Part print with two shaded views. Sizes in mm from the minimum x, y, z corner. A direction names the side the tool comes from. Coordinates: 2 decimals unless noted, no trailing zeros. Order: outer loops, then holes, each group sorted by start corner. A loop starts at its lowest first (then second) coordinate and runs counter-clockwise, first axis right, second up.
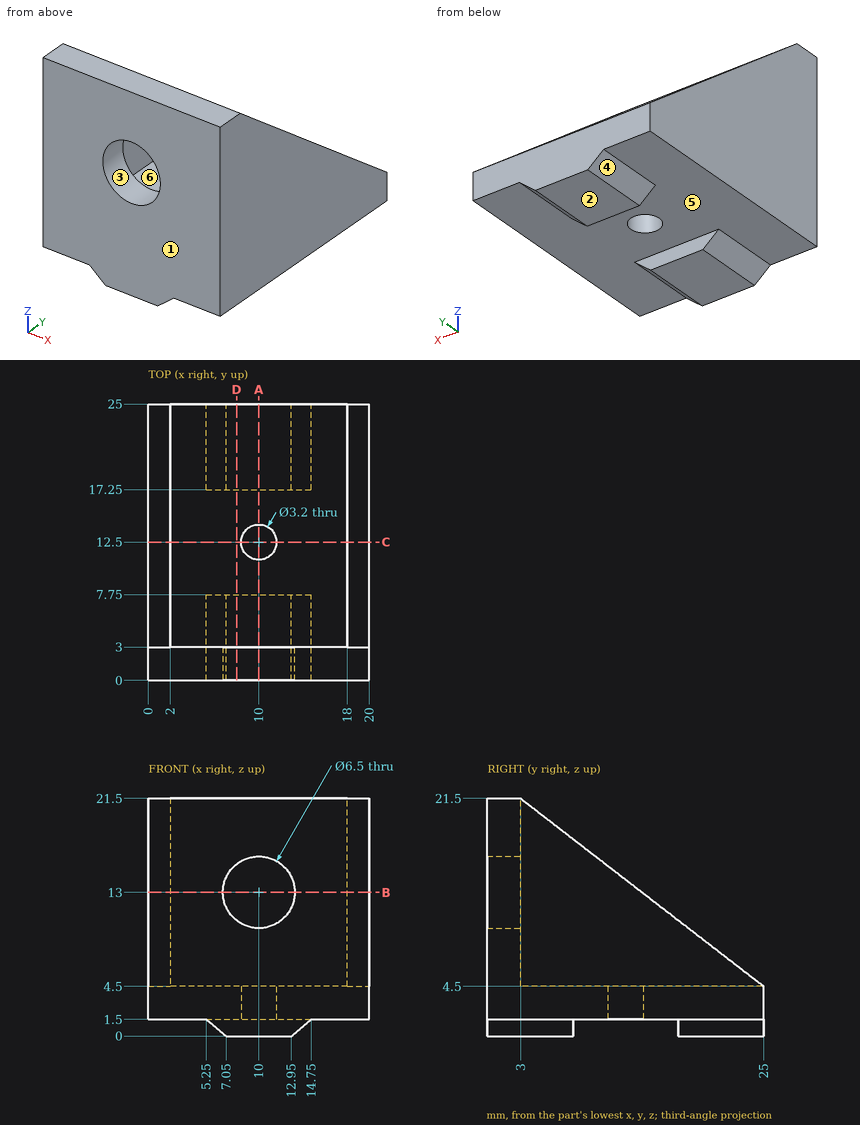
Q1. Pin check, flat tips, straight feed: pin 1 Ø3 at (x, z) = (2, 8.5) entering from -Y; pin 2 Ø8 at (x, y) = (16.5, 11) entering from +Z; pin 3 Ø1.5 at (x, y) = (4, 20) entering from -Z; pin 4 Ø6 at (x, z) = (10, 13) entering from +Y. Stop position of each tip, or through.
Results list:
pin 1: stops at y = 0
pin 2: stops at z = 18.18
pin 3: stops at z = 1.5
pin 4: passes through
Q2. Cut at D-D on x = 8. Write the cut outline in (y, z), and give its area (3 significant figures).
Results list:
outline: (0, 0) - (7.75, 0) - (7.75, 1.5) - (17.25, 1.5) - (17.25, 0) - (25, 0) - (25, 4.5) - (3, 4.5) - (3, 10.44) - (0, 10.44) - close; (0, 15.56) - (3, 15.56) - (3, 21.5) - (0, 21.5) - close
area: 134 mm2
Q3. Cut at B-B on z = 13. Write the cut outline in (x, y).
Results list:
outline: (0, 0) - (6.75, 0) - (6.75, 3) - (2, 3) - (2, 14) - (0, 14) - close; (13.25, 0) - (20, 0) - (20, 14) - (18, 14) - (18, 3) - (13.25, 3) - close
Q4. Wall check: line 1 along Z through (x, y) = (10, 0.95); line 2 along X through (y, z) = (7, 9.25); line 3 along X through (y, z) = (12.5, 3.6). Give the ranges that are in metal, low to high.
Results list:
line 1: z = 0 to 9.75, 16.25 to 21.5
line 2: x = 0 to 2, 18 to 20
line 3: x = 0 to 8.4, 11.6 to 20
Q5. Cut at A-A on x = 10. Write the cut outline in (y, z).
Results list:
outline: (0, 0) - (7.75, 0) - (7.75, 1.5) - (10.9, 1.5) - (10.9, 4.5) - (3, 4.5) - (3, 9.75) - (0, 9.75) - close; (0, 16.25) - (3, 16.25) - (3, 21.5) - (0, 21.5) - close; (14.1, 1.5) - (17.25, 1.5) - (17.25, 0) - (25, 0) - (25, 4.5) - (14.1, 4.5) - close
Q6. Cut at C-C on y = 12.5. Write the cut outline in (x, z).
Results list:
outline: (0, 1.5) - (8.4, 1.5) - (8.4, 4.5) - (2, 4.5) - (2, 14.16) - (0, 14.16) - close; (11.6, 1.5) - (20, 1.5) - (20, 14.16) - (18, 14.16) - (18, 4.5) - (11.6, 4.5) - close
Q7. Which spindle directions (+Z, -Z, +X, -X, +Y, -Y) get a long thin tool onto all of the face, cutting with end or side? Do the marked faces 4, 5 and 6. Say none if no direction does.
Results list:
face 4: -Z, -X, +Y, -Y
face 5: -Z
face 6: +Z, +Y
Q8. Mould opens along Z. For the marked faces 1, 2 and 3 say: pulls with the +Z half, pulls with the -Z half, needs draft (parallel to the pull), parting line crosses it, or undercut.
Results list:
face 1: needs draft
face 2: pulls with the -Z half
face 3: undercut
